Job drawing, mm, ordinate dimensions from the low corner. One solid piece. Give positions to 0.01 mm unless a question says otherwise; leave off trailing zeros. Write each loop counter-clockwise with the first axis right and the second up, starting at its lowest first coordinate (ties: lowest second). Pieces come first, ordered by that corner, then holes. Notation, with made-up numbers: (-13.75, -4) -> (34.25, -4) arc R8 cw to (34.25, 0) -> close; hole circle Ø1 at (-12, 48). An arc over 180 degrees is marked (long way). Put each result on its own line as item: value. Start each with the question number.
Item 1: Slice it at B-B, the plane y = 3.25. List the corners of the cut face in (x, z).
Item 2: Two-plate mould, pull along X, no slides. Class the marked faces 1, 2 and 3: pulls with the +X half, pulls with the -X half, needs draft (parallel to the pull), parting line crosses it, or undercut.
Item 3: Slice it at A-A, the plane x = 29. List the corners of the cut face in (y, z).
Item 4: Slice it at C-C, the plane y = 15. List the corners of the cut face in (x, z), plus the area to 3 significant figures.
Item 5: Flat gauge pins, fed straight in: pin 1 Ø3 at (x, z) = (22.5, 35.5) entering from -Y; pin 2 Ø3 at (x, z) = (43.5, 49) entering from -Y; pin 3 Ø3 at (x, y) = (42, 8.5) entering from +Z. Where does each tip first touch, or does it go through?
Item 6: Drill centre lines: line 1 along X through (y, z) = (2.5, 29); line 2 along X through (y, z) = (2.75, 19.5); line 3 along Y through (x, z) = (33.5, 23). Where is each one in solid material? Low to high.
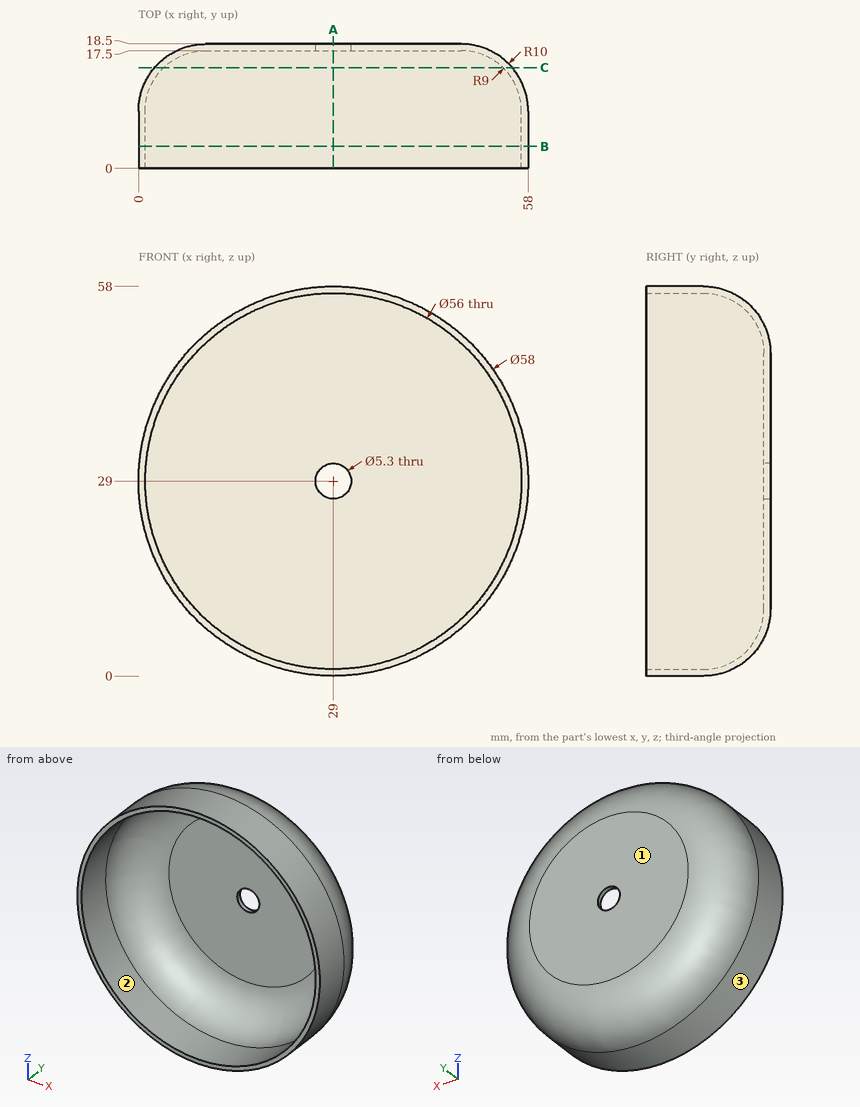
Values follow:
1. outline: circle Ø58 at (29, 29); hole circle Ø56 at (29, 29)
2. face 1: needs draft
2. face 2: undercut
2. face 3: parting line crosses it
3. outline: (0, 0) -> (8.5, 0) arc R10 ccw to (18.5, 10) -> (18.5, 26.35) -> (17.5, 26.35) -> (17.5, 10) arc R9 cw to (8.5, 1) -> (0, 1) -> close; (0, 57) -> (8.5, 57) arc R9 cw to (17.5, 48) -> (17.5, 31.65) -> (18.5, 31.65) -> (18.5, 48) arc R10 ccw to (8.5, 58) -> (0, 58) -> close
4. outline: circle Ø53.2 at (29, 29); hole circle Ø50.45 at (29, 29)
4. area: 224 mm2
5. pin 1: y = 17.5
5. pin 2: y = 13.9
5. pin 3: z = 55.62
6. line 1: 0 to 1, 57 to 58
6. line 2: 1.6 to 2.66, 55.34 to 56.4
6. line 3: 17.5 to 18.5
